Can you work these out from the model? Positions are in its coordinate system, mm. A direction names the side the tool comes from. Give positions to 0.01 mm unless a question says otherwise; leave off trailing zeros. Write each loop counter-clockwise with the first axis right and the second up, starting at its lowest first coordinate (ties: lowest second). Pieces come first, ordered by that corner, then holes.
from build123d import *

# Parameters (mm, degrees)
CROQUIS1_R              = 200
SALIENTE_EXTRUIR1_DEPTH = 900
REDONDEO1_R             = 90
CROQUIS2_R              = 60
SALIENTE_EXTRUIR2_DEPTH = 90
CROQUIS3_W              = 120
CROQUIS3_H              = 90.836251912
SALIENTE_EXTRUIR3_DEPTH = 60
SALIENTE_EXTRUIR4_DEPTH = 90.836252
CROQUIS5_W              = 120
CROQUIS5_H              = 90.836251912
SALIENTE_EXTRUIR5_DEPTH = 60
SALIENTE_EXTRUIR6_DEPTH = 90.836252
REDONDEO2_R             = 8
CROQUIS8_R              = 45.418125956
SALIENTE_EXTRUIR7_DEPTH = 30
CROQUIS9_R              = 32.5
CROQUIS10_R             = 32.5
SALIENTE_EXTRUIR8_DEPTH = 50
SALIENTE_EXTRUIR8_TAPER = 11


with BuildPart() as part:
    # Croquis1 → Saliente-Extruir1 (new body)
    with BuildSketch(Plane(origin=(0, 0, 0), x_dir=(1, 0, 0), z_dir=(0, 1, 0))):
        Circle(CROQUIS1_R)
    extrude(amount=SALIENTE_EXTRUIR1_DEPTH)

    # Redondeo1
    redondeo1_edges = [part.edges().sort_by_distance(p)[0] for p in [
        (-200, 900, 0),
    ]]
    fillet(redondeo1_edges, radius=REDONDEO1_R)

    # Croquis2 → Saliente-Extruir2 (add)
    with BuildSketch(Plane(origin=(0, 900, 0), x_dir=(1, 0, 0), z_dir=(0, 1, 0))):
        Circle(CROQUIS2_R)
    extrude(amount=SALIENTE_EXTRUIR2_DEPTH)

    # Croquis3 → Saliente-Extruir3 (add)
    with BuildSketch(Plane(origin=(0, 990, 0), x_dir=(1, 0, 0), z_dir=(0, 1, 0))):
        Rectangle(CROQUIS3_W, CROQUIS3_H)
    extrude(amount=SALIENTE_EXTRUIR3_DEPTH)

    # Croquis4 → Saliente-Extruir4 (add)
    with BuildSketch(Plane.XY.offset(45.418125956)):
        with BuildLine():
            Line((60, 990), (432.304083803, 829.898605595))
            Line((432.304083803, 829.898605595), (442.878538819, 854.488727381))
            ThreePointArc((442.878538819, 854.488727381), (259.713592606, 968.448343813), (60, 1050))
            Line((60, 1050), (60, 990))
        make_face()
    extrude(amount=-SALIENTE_EXTRUIR4_DEPTH)

    # Croquis5 → Saliente-Extruir5 (add)
    with BuildSketch(Plane(origin=(0, 1050, 0), x_dir=(1, 0, 0), z_dir=(0, 1, 0))):
        Rectangle(CROQUIS5_W, CROQUIS5_H)
    extrude(amount=SALIENTE_EXTRUIR5_DEPTH)

    # Croquis6 → Saliente-Extruir6 (add)
    with BuildSketch(Plane.XY.offset(45.418125956)):
        with BuildLine():
            Line((346.814814122, 1222.018811659), (368.82653308, 1180.746838612))
            ThreePointArc((368.82653308, 1180.746838612), (207.813070235, 1130.963209195), (60, 1050))
            Line((60, 1050), (60, 1110))
            Line((60, 1110), (32.230664011, 1110))
            ThreePointArc((32.230664011, 1110), (182.778174474, 1184.950270214), (346.814814122, 1222.018811659))
        make_face()
    extrude(amount=-SALIENTE_EXTRUIR6_DEPTH)

    # Redondeo2
    redondeo2_edges = [part.edges().sort_by_distance(p)[0] for p in [
        (246.152041901, 909.949302798, 45.418125956),
        (259.713592606, 968.448343813, 45.418125956),
        (259.713592606, 968.448343813, -45.418126044),
        (246.152041901, 909.949302798, -45.418126044),
        (207.813070235, 1130.963209195, 45.418125956),
        (182.778174474, 1184.950270214, 45.418125956),
        (207.813070235, 1130.963209195, -45.418126044),
        (182.778174474, 1184.950270214, -45.418126044),
    ]]
    fillet(redondeo2_edges, radius=REDONDEO2_R)

    # Croquis8 → Saliente-Extruir7 (add)
    with BuildSketch(Plane.ZY.offset(60)):
        with Locations((0, 1050)):
            Circle(CROQUIS8_R)
    extrude(amount=SALIENTE_EXTRUIR7_DEPTH)

    # Barrer1: sweep along a curve in space
    with BuildLine() as barrer1_path:
        Line((-90, 1050, 0), (-120, 1050, 0))
        ThreePointArc((-120, 1050, 0), (-240.208152802, 1000.208152802, 0), (-290, 880, 0))
        Line((-290, 880, 0), (-290, 150, 0))
    # Croquis9 → Barrer1 (sweep)
    with BuildSketch(Plane.ZY.offset(90)):
        with Locations((0, 1050)):
            Circle(CROQUIS9_R)
    sweep(path=barrer1_path.line)

    # Croquis10 → Saliente-Extruir8 (add)
    with BuildSketch(Plane.XZ.offset(-150)):
        with Locations((-290, 0)):
            Circle(CROQUIS10_R)
    extrude(amount=SALIENTE_EXTRUIR8_DEPTH, taper=SALIENTE_EXTRUIR8_TAPER)


solid = part.part
(1) For faces 4 (the face through (-59.94, 944.37, -2.64)), 5 (the face through (243.55, 911.07, 0.52)), 6 (the face through (135, 1013, -45.418)), which set-ups out of +Z, -Z, +X, -X, +Y, -Y let a thin tool reach every point of the face, with its end or its side?
Returned:
face 4: none
face 5: +Z, -Z
face 6: -Z, +X, +Y
(2) Will these pins go through, and if not, where does the flat tip stop? P1, Ø4, axis at x = -15.5, y = 376.5, coming from the -Z side; P2, Ø3, axis at x = 8, y = 370.5, coming from the +Z side; P3, Ø5, axis at y = 464, z = -143, coming from the -X side.
Returned:
P1: stops at z = -199.54
P2: stops at z = 199.89
P3: stops at x = -142.34
(3) If we mould it in two halves opening along Y, with no side actions, what happens to faces 1 (the face through (-265.53, 119.09, -10.15)), 2 (the face through (-90, 1081, -11)), 3 (the face through (-60, 1100, 1))? For each: +Y half, -Y half, draft (parallel to the pull), parting line (faces both ways), or undercut.
Returned:
face 1: -Y half
face 2: undercut
face 3: draft
(4) Imagine slicing it at A-A, the plane x = 0. Write out the boundary of the cut face in (y, z), plus the area to 3 significant figures.
Returned:
outline: (0, -200) - (810, -200) arc R90 ccw to (900, -110) - (900, -60) - (990, -60) - (990, -45.42) - (1110, -45.42) - (1110, 45.42) - (990, 45.42) - (990, 60) - (900, 60) - (900, 110) arc R90 ccw to (810, 200) - (0, 200) - close
area: 378,000 mm2
(5) Imagine slicing it at C-C, the plane y = 970. Give the number of separate pieces and of enclosed holes in the cut face, plus the area to 3 significant figures.
Returned:
separate pieces: 3
enclosed holes: 0
area: 28,800 mm2
(6) If I drill on L1, parallel to Y at x = -54.5, z = 77.5; L2, parallel to Z at x = -33, y = 1094; L3, parallel to X at y = 963, z = -29, over which ranges is the centre line in solid material (lowest first)?
Returned:
L1: y = 0 to 900
L2: z = -45.42 to 45.42
L3: x = -284.97 to -251.29, -52.53 to 52.53, 122.79 to 270.26
(7) Imagine slicing it at B-B, the plane y = 730. Write out the boundary of the cut face in (x, z), plus the area to 3 significant figures.
Returned:
outline: circle Ø65 at (-290, 0); circle Ø400 at (0, 0)
area: 129,000 mm2
